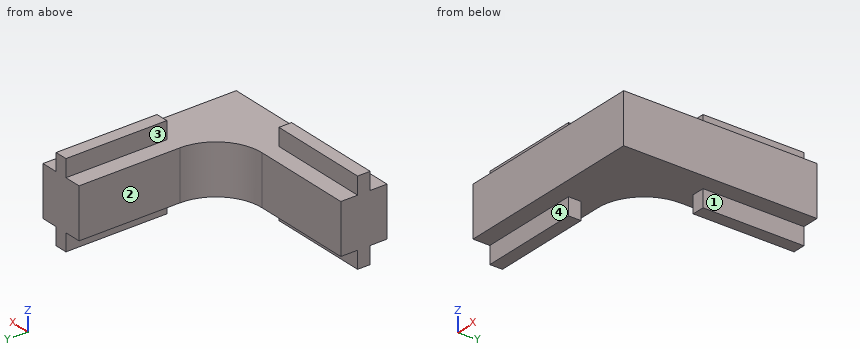
from build123d import *

# Parameters (mm, degrees)
BOSS_EXTRUDE1_DEPTH = 5.9
SKETCH2_W           = 12
SKETCH2_H           = 1.5
SKETCH2_W_2         = 1.5
SKETCH2_H_2         = 12
BOSS_EXTRUDE2_DEPTH = 2.05


with BuildPart() as part:
    # Sketch1 → Boss-Extrude1 (new body)
    with BuildSketch(Plane.XY):
        with BuildLine():
            Line((0, 5.5), (12, 5.5))
            ThreePointArc((12, 5.5), (15.889087297, 7.110912703), (17.5, 11))
            Line((17.5, 11), (17.5, 23))
            Line((17.5, 23), (23, 23))
            Line((23, 23), (23, 0))
            Line((23, 0), (0, 0))
            Line((0, 0), (0, 5.5))
        make_face()
    extrude(amount=BOSS_EXTRUDE1_DEPTH)

    # Sketch2 → Boss-Extrude2 (add)
    with BuildSketch(Plane.XY.offset(5.9)):
        with Locations((6, 2.75)):
            Rectangle(SKETCH2_W, SKETCH2_H)
        with Locations((20.25, 17)):
            Rectangle(SKETCH2_W_2, SKETCH2_H_2)
    boss_extrude2 = extrude(amount=BOSS_EXTRUDE2_DEPTH)

    # Mirror1: Boss-Extrude2 across plane
    add(boss_extrude2.mirror(Plane.XY.offset(2.95)))


solid = part.part
Check sheet for the modelled part. Datum: model origin and axes. Units: mm. Face numbers are marked on the shaded views. A direction names the side the tool comes from. Give positions to 0.01 mm unless a question says otherwise; leave off trailing zeros. Loops run counter-clockwise (first coordinate to the right, second up) from the corner with the lowest first, then second, coordinate; pieces in that order, holes last. Notation, with made-up numbers: M -21.5,29.5 L 34.5,29.5 A16 cw 34.5,56.5 Z; hole C 13,19.5 d6. An arc over 180 degrees is marked long. Return JSON: item names as keys, results as strings. Group by question number.
1. Go/stop test with flat-tipped pins: pin 1 (10 mm diameter, centred on x = 11, y = 13.5, fed in from -Z); pin 2 (1.2 mm diameter, centred on x = 20.5, z = -1, fed in from -Y); pin 3 (1.5 mm diameter, centred on y = 14.5, z = -0.5, fed in from -X); pin 4 (1.6 mm diameter, centred on x = 4.5, z = -0.5, fed in from +Y). Record where each tip stops, or that it passes through.
2. Thickness scan on L1, parallel to Z at x = 19, y = 1.75; L2, parallel to Y at x = 5.5, z = 3.5; L3, parallel to Y at x = 20.5, z = -0.5. Record the ranges inside material, lowest first.
3. Cross-section at B-B on x = 4. Record the boundary of the cut face in (y, z).
4. Cross-section at A-A on z = -0.75. Record the boundary of the cut face in (x, y).
5. Cross-section at D-D on z = 5. Record the boundary of the cut face in (x, y).
6. Cross-section at C-C on y = 13. Record the boundary of the cut face in (x, z), plus the area to 3 significant figures.
7. Tool access check on the marked faces 1, 2, 3 and 4. Record the directions out of +Z, -Z, +X, -X, +Y, -Y that give a thin tool (end or side, any length) a straight path to the whole face; none if there is none.
Return value:
{
 "1": {"pin 1": "through", "pin 2": "y = 11", "pin 3": "x = 17.5", "pin 4": "y = 5.5"},
 "2": {"L1": "0 to 5.9", "L2": "0 to 5.5", "L3": "11 to 23"},
 "3": {"outline": "M 0,0 L 2,0 L 2,-2.05 L 3.5,-2.05 L 3.5,0 L 5.5,0 L 5.5,5.9 L 3.5,5.9 L 3.5,7.95 L 2,7.95 L 2,5.9 L 0,5.9 Z"},
 "4": {"outline": "M 0,2 L 12,2 L 12,3.5 L 0,3.5 Z; M 19.5,11 L 21,11 L 21,23 L 19.5,23 Z"},
 "5": {"outline": "M 0,0 L 23,0 L 23,23 L 17.5,23 L 17.5,11 A5.5 cw 12,5.5 L 0,5.5 Z"},
 "6": {"outline": "M 17.5,0 L 19.5,0 L 19.5,-2.05 L 21,-2.05 L 21,0 L 23,0 L 23,5.9 L 21,5.9 L 21,7.95 L 19.5,7.95 L 19.5,5.9 L 17.5,5.9 Z", "area": "38.6 mm^2"},
 "7": {"face 1": "-Z, +X, +Y, -Y", "face 2": "+Z, -Z, -X, +Y", "face 3": "+Z, -X, +Y, -Y", "face 4": "-Z, +X, -X, -Y"}
}
